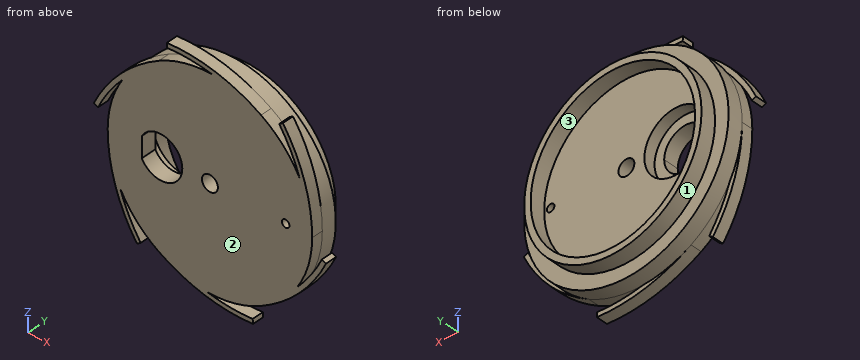
from build123d import *

# Parameters (mm, degrees)
BOSS_EXTRUDE1_DEPTH        = 3
F_4_2_4_2_DIAMETER_HOLE1_D = 4.2
SKETCH24_R                 = 1
CUT_EXTRUDE3_DEPTH         = 10
SKETCH25_R                 = 8.25
CUT_EXTRUDE4_DEPTH         = 3


with BuildPart() as part:
    # Sketch1 → Revolve1 (revolve)
    with BuildSketch(Plane.XY):
        Polygon((-23.425, 0), (-23.425, -4), (-27, -4), (-27, -8), (0, -8), (0, -4), (-21.721500416, -4), (-21.721500416, 0), align=None)
    revolve(axis=Axis((0, -8, 0), (0, -1, 0)))

    # Sketch18 → Boss-Extrude1 (add)
    with BuildSketch(Plane.XZ.offset(8)):
        with BuildLine():
            Line((18.287619048, 23.591829478), (19.266666667, 24.285706816))
            ThreePointArc((19.266666667, 24.285706816), (25.019995002, 12.743625858), (27, 0))
            ThreePointArc((27, 0), (25.997622732, -7.288594671), (23.06491761, -14.036009962))
            ThreePointArc((23.06491761, -14.036009962), (26.687121428, -9.277998508), (29.574933174, -4.041627931))
            Line((29.574933174, -4.041627931), (30.665372385, -4.542569372))
            ThreePointArc((30.665372385, -4.542569372), (23.54630123, -15.296138346), (13.5, -23.382685902))
            ThreePointArc((13.5, -23.382685902), (6.686703224, -26.158899059), (-0.62308239, -26.992809567))
            ThreePointArc((-0.62308239, -26.992809567), (5.30857831, -27.750724365), (11.287314126, -27.633457409))
            Line((11.287314126, -27.633457409), (11.398705718, -28.828276188))
            ThreePointArc((11.398705718, -28.828276188), (-1.473693772, -28.039764204), (-13.5, -23.382685902))
            ThreePointArc((-13.5, -23.382685902), (-19.310919509, -18.870304389), (-23.688, -12.956799605))
            ThreePointArc((-23.688, -12.956799605), (-21.378543119, -18.472725857), (-18.287619048, -23.591829478))
            Line((-18.287619048, -23.591829478), (-19.266666667, -24.285706816))
            ThreePointArc((-19.266666667, -24.285706816), (-25.019995002, -12.743625858), (-27, 0))
            ThreePointArc((-27, 0), (-25.997622732, 7.288594671), (-23.06491761, 14.036009962))
            ThreePointArc((-23.06491761, 14.036009962), (-26.687121428, 9.277998508), (-29.574933174, 4.041627931))
            Line((-29.574933174, 4.041627931), (-30.665372385, 4.542569372))
            ThreePointArc((-30.665372385, 4.542569372), (-23.54630123, 15.296138346), (-13.5, 23.382685902))
            ThreePointArc((-13.5, 23.382685902), (-6.686703224, 26.158899059), (0.62308239, 26.992809567))
            ThreePointArc((0.62308239, 26.992809567), (-5.30857831, 27.750724365), (-11.287314126, 27.633457409))
            Line((-11.287314126, 27.633457409), (-11.398705718, 28.828276188))
            ThreePointArc((-11.398705718, 28.828276188), (1.473693772, 28.039764204), (13.5, 23.382685902))
            ThreePointArc((13.5, 23.382685902), (19.310919509, 18.870304389), (23.688, 12.956799605))
            ThreePointArc((23.688, 12.956799605), (21.378543119, 18.472725857), (18.287619048, 23.591829478))
        make_face()
    extrude(amount=BOSS_EXTRUDE1_DEPTH)

    # Ø4.2 (4.2) Diameter Hole1 (through all)
    with Locations(Plane(origin=(0, -4, 0), x_dir=(1, 0, 0), z_dir=(0, 1, 0))):
        with Locations((0, 0)):
            Hole(F_4_2_4_2_DIAMETER_HOLE1_D / 2)

    # Sketch24 → Cut-Extrude3 (cut)
    with BuildSketch(Plane.XZ.offset(11)):
        with BuildLine():
            ThreePointArc((-7.3, 0), (-11.587555311, 5.522227811), (-18, 2.736786437))
            Line((-18, 2.736786437), (-18, -2.736786437))
            ThreePointArc((-18, -2.736786437), (-11.587555311, -5.522227811), (-7.3, 0))
        make_face()
        with Locations((20, 0)):
            Circle(SKETCH24_R)
    extrude(amount=-CUT_EXTRUDE3_DEPTH, mode=Mode.SUBTRACT)

    # Sketch25 → Cut-Extrude4 (cut)
    with BuildSketch(Plane(origin=(0, -4, 0), x_dir=(1, 0, 0), z_dir=(0, 1, 0))):
        with Locations((-13, 0)):
            Circle(SKETCH25_R)
    extrude(amount=-CUT_EXTRUDE4_DEPTH, mode=Mode.SUBTRACT)


solid = part.part
Work out the finished part from the listing and answer in its coordinate system (mm). Face numbers are marked on the shaded views. Give positions to 0.01 mm unless a question says otherwise; leave off trailing zeros. Loops run counter-clockwise (first coordinate to the right, second up) from the corner with the lowest first, then second, coordinate; pieces in that order, holes last. Notation, with made-up numbers: (2.25, 26) - (7.25, 26) arc R32 ccw to (7.25, 65) - close; hole circle Ø6 at (8.5, -4.5). An arc over 180 degrees is marked (long way). Answer in a Markdown table with one row per item. Add a question column.
Q1. Consider line 1 along X through (y, z) = (-3.75, -0.5); line 2 along Z through (x, y) = (0, -1.45) (1 decimal); line 3 along Z through (x, y) = (20, -8.5). Determine where each line is inside the solid, lowest interval first.
Q2. The part is cut by section C-C (x = 3.5). Determine the outline of the cut face in (y, z), and give its area (3 significant figures).
Q3. Each of these flat-tipped pins is pushed along its axis until it touches: P1, Ø1, axis at x = -1.5, z = 1, coming from the -Y side; P2, Ø16, axis at x = 5.5, z = -4.5, coming from the +Y side; P3, Ø1.5, axis at x = 19, y = -9, coming from the +Z side; P4, Ø4, axis at x = 22, y = -5.5, coming from the +Z side. Where does it stop, or does it pass through?
Q4. Determine the mould class of the marked faces 1, 2 and 3 for opening direction Z: released by +Z, released by -Z, zero draft, split by the parting line, or undercut.
Q5. The part is cut by section B-B (x = 20). Determine the outline of the cut face in (y, z).
Q6. The part is cut by section A-A (z = 9.5). Determine the outline of the cut face in (x, y).
Solution:
| question | item | result |
|---|---|---|
| 1 | line 1 | x = -23.42 to -21.72, 21.72 to 23.42 |
| 1 | line 2 | z = -23.4 to -21.7, 21.7 to 23.4 |
| 1 | line 3 | z = -18.75 to -1, 1 to 18.14, 20.97 to 23.22 |
| 2 | outline | (-11, -28.82) - (-8, -28.82) - (-8, -27.61) - (-11, -27.61) - close; (-11, -26.77) - (-4, -26.77) - (-4, -23.16) - (0, -23.16) - (0, -21.44) - (-4, -21.44) - (-4, 21.44) - (0, 21.44) - (0, 23.16) - (-4, 23.16) - (-4, 26.77) - (-8, 26.77) - (-8, 27.54) - (-11, 27.54) - close |
| 2 | area | 395 mm² |
| 3 | P1 | stops at y = -11 |
| 3 | P2 | stops at y = -4 |
| 3 | P3 | stops at z = 24.29 |
| 3 | P4 | stops at z = 18.14 |
| 4 | face 1 | split by the parting line |
| 4 | face 2 | zero draft |
| 4 | face 3 | undercut |
| 5 | outline | (-11, -18.75) - (-8, -18.75) - (-8, -18.14) - (-4, -18.14) - (-4, -12.2) - (0, -12.2) - (0, -8.47) - (-4, -8.47) - (-4, -1) - (-11, -1) - close; (-11, 1) - (-4, 1) - (-4, 8.47) - (0, 8.47) - (0, 12.2) - (-4, 12.2) - (-4, 18.14) - (-11, 18.14) - close; (-11, 20.97) - (-8, 20.97) - (-8, 23.22) - (-11, 23.22) - close |
| 6 | outline | (-27.97, -11) - (-26.54, -11) - (-26.54, -8) - (-27.97, -8) - close; (-25.27, -11) - (25.91, -11) - (25.91, -8) - (25.27, -8) - (25.27, -4) - (21.41, -4) - (21.41, 0) - (19.53, 0) - (19.53, -4) - (-19.53, -4) - (-19.53, 0) - (-21.41, 0) - (-21.41, -4) - (-25.27, -4) - close |
